The listing builds one solid part. Answer for the finished solid, in the listing's coordinates (mm). A direction names the side the tool comes from. Coordinates: 2 decimals unless noted, no trailing zeros. Order: outer loops, then holes, each group sorted by start corner. A loop starts at its lowest first (then second) coordinate and runs counter-clockwise, first axis right, second up. Notation, with made-up numbers: (4.5, 64.5) -> (27.5, 64.5) arc R22 ccw to (27.5, 98.5) -> close; hole circle Ø11 at (68.25, 68). An arc over 180 degrees is marked (long way). Write each question's results on one line, items separated by ' | '. Start each with the question number.
(1) Straight lines are drawn through the part: L1, parallel to X at y = 6, z = 6; L2, parallel to Y at x = 8.75, z = 13.25; L3, parallel to X at y = -4, z = 2. For each, find the intervals that lie inside material, in ascending order.
(2) Determine the mould class of faces 1 (the face through (3, -6.5, 0)), 2 (the face through (0, -8, 7)), 3 (the face through (13, 0, 11)) for opening direction Y: +Y half, -Y half, draft (parallel to the pull), parting line (faces both ways), or undercut.
(3) The part is cut by section C-C, the plane x = -7.5. Give the vertices of the cut face in (y, z), then the cut area to 3 significant figures.
(4) The part is cut by section B-B, the plane y = 4.25. Give the vertices of the cut face in (x, z), then the cut area to 4 significant figures.
(5) The part is cut by section A-A, the plane z = 13. Give the vertices of the cut face in (x, y), then the cut area to 3 significant figures.
(6) Given pin 1 (1 mm diameter, centred on x = 13.5, y = -0.5, fed in from +Z); pin 2 (5 mm diameter, centred on x = -4, y = -5, fed in from +Z); pin 3 (0.6 mm diameter, centred on x = -13, y = -2.5, fed in from -Z), each flat-ended and moving along its own axis, determine where each tip first touches the part or whether it passes through.
(7) The part is cut by section D-D, the plane z = 6.5. Give the vertices of the cut face in (x, y), then the cut area to 3 significant figures.
(8) A tool of negligible diameter and unlimited length cuts with its end or side. For faces 4 (the face through (-0.2, 6.4, 15)), 5 (the face through (-12.05, 0, 10)), 6 (the face through (-13, 0, 5)), 7 (the face through (-13, 0, 11)), 8 (the face through (14, 0, 7)), from which of +Z, -Z, +X, -X, +Y, -Y can it reach the whole face along a straight path? Write none if from no direction.
```python
from build123d import *

# Parameters (mm, degrees)
SKETCH013_W     = 28
SKETCH013_H     = 16
SKETCH013_W_2   = 24.1
SKETCH013_H_2   = 12.1
PAD004_DEPTH    = 15
SKETCH014_W     = 30
SKETCH014_H     = 4
POCKET010_DEPTH = 4
SKETCH015_W     = 12.1
SKETCH015_H     = 5
POCKET011_DEPTH = 5


with BuildPart() as part:
    # Sketch013 → Pad004 (new body)
    with BuildSketch(Plane.XY):
        Rectangle(SKETCH013_W, SKETCH013_H)
        Rectangle(SKETCH013_W_2, SKETCH013_H_2, mode=Mode.SUBTRACT)
    extrude(amount=PAD004_DEPTH)

    # Sketch014 → Pocket010 (cut)
    with BuildSketch(Plane.XY.offset(15)):
        Rectangle(SKETCH014_W, SKETCH014_H)
    extrude(amount=-POCKET010_DEPTH, mode=Mode.SUBTRACT)

    # Sketch015 → Pocket011 (cut)
    with BuildSketch(Plane(origin=(-14, 0, 0), x_dir=(0, -1, 0), z_dir=(-1, 0, 0))):
        with Locations((0, 2.5)):
            Rectangle(SKETCH015_W, SKETCH015_H)
    extrude(amount=-POCKET011_DEPTH, mode=Mode.SUBTRACT)


solid = part.part
```
Established:
1) L1: x = -14 to -12.05, 12.05 to 14 | L2: y = -8 to -6.05, 6.05 to 8 | L3: x = 12.05 to 14
2) face 1: draft | face 2: -Y half | face 3: undercut
3) outline: (-8, 0) -> (-6.05, 0) -> (-6.05, 15) -> (-8, 15) -> close; (6.05, 0) -> (8, 0) -> (8, 15) -> (6.05, 15) -> close | area: 58.5 mm^2
4) outline: (-14, 5) -> (-12.05, 5) -> (-12.05, 15) -> (-14, 15) -> close; (12.05, 0) -> (14, 0) -> (14, 15) -> (12.05, 15) -> close | area: 48.75 mm^2
5) outline: (-14, -8) -> (14, -8) -> (14, -2) -> (12.05, -2) -> (12.05, -6.05) -> (-12.05, -6.05) -> (-12.05, -2) -> (-14, -2) -> close; (-14, 2) -> (-12.05, 2) -> (-12.05, 6.05) -> (12.05, 6.05) -> (12.05, 2) -> (14, 2) -> (14, 8) -> (-14, 8) -> close | area: 141 mm^2
6) pin 1: stops at z = 11 | pin 2: stops at z = 15 | pin 3: stops at z = 5
7) outline: (-14, -8) -> (14, -8) -> (14, 8) -> (-14, 8) -> close; hole (-12.05, -6.05) -> (12.05, -6.05) -> (12.05, 6.05) -> (-12.05, 6.05) -> close | area: 156 mm^2
8) face 4: +Z, +X, -X, +Y, -Y | face 5: +Z, -Z | face 6: -Z, -X | face 7: +Z, +X, -X | face 8: +Z, -Z, +X, +Y, -Y
